from build123d import *

# Parameters (mm, degrees)
F1_DEPTH = 6.35
F0_W     = 265.508406
F0_H     = 162.831157
F2_DEPTH = 5.08


with BuildPart() as f1:
    # F0 (on Front) → F1 (new body, symmetric)
    with BuildSketch(Plane.XZ):
        with BuildLine():
            ThreePointArc((-20.447047, -1.391527), (0, -51.461593), (20.447047, -1.391527))
            ThreePointArc((20.447047, -1.391527), (0, 39.077588), (-20.447047, -1.391527))
        make_face()
        with BuildLine():
            ThreePointArc((15.056898, -1.795547), (0, -47.651593), (-15.056898, -1.795547))
            ThreePointArc((-15.056898, -1.795547), (0, 35.267588), (15.056898, -1.795547))
        make_face(mode=Mode.SUBTRACT)
    extrude(amount=F1_DEPTH, both=True)

    # F0 (on Front) → F2 (join, symmetric)
    with BuildSketch(Plane.XZ):
        with Locations((11.139218, -0.917264)):
            Rectangle(F0_W, F0_H)
        with BuildLine():
            ThreePointArc((-20.447047, -1.391527), (0, 39.077588), (20.447047, -1.391527))
            ThreePointArc((20.447047, -1.391527), (0, -51.461593), (-20.447047, -1.391527))
        make_face(mode=Mode.SUBTRACT)
    extrude(amount=F2_DEPTH, both=True)


solid = f1.part
Input: part model. Units: mm. Frame: model coordinates. A direction names the side the tool comes from. Give positions to 0.01 mm unless a question says otherwise; leave off trailing zeros. Write each loop counter-clockwise with the first axis right and the second up, starting at its lowest first coordinate (ties: lowest second). Pieces come first, ordered by that corner, then holes. Notation, with made-up numbers: M 60.25,-34.75 L 73.25,-34.75 A4 ccw 73.25,-30.75 Z; hole C -9,-33 d9. An arc over 180 degrees is marked long. Write item = value, one per line. Start each with the question number.
1) Reachability of faces 1 (the flat face through (9, 0, -82.333)), 2 (the cylindrical face through (0.784, -5.724, 39.065)), 3 (the cylindrical face through (-0.967, 5.706, -51.446)) from +Z, -Z, +X, -X, +Y, -Y: full face, straight path, thin tool, end or side. Return the list, or none.
2) First-contact query: pin 1 Ø8 at (x, z) = (-76, 22) entering from +Y. Flat tip, straight axial feed; report the tip coordinate or a pass-through.
3) Cut plane D-D on x = -56.5. Return the cut outline in (y, z), then the cut area to 3 significant figures.
4) Material intervals for line 1 along Z through (x, y) = (0, -1.25); line 2 along X through (y, z) = (-5.25, 13); line 3 along Y through (x, z) = (65, 60), sorted ascending. Write a range as [from, to].
5) Draft query along Z for faces 4 (the cylindrical face through (0.784, 5.706, 39.065)), 5 (the cylindrical face through (0.891, -0.089, -47.636)), 6 (the flat face through (-17, 6.35, -3)), 7 (the flat face through (9, 0, 80.498)). Return one class per face: +Z half, -Z half, draft (parallel to the pull), parting line (faces both ways), or undercut.
6) Cut plane C-C on y = -3. Return the cut outline in (x, z), then the cut area to 3 significant figures.
7) Cut plane B-B on z = 25. Return the cut outline in (x, y), then the cut area to 3 significant figures.
8) Cut plane A-A on x = 0. Return the cut outline in (y, z).
Solved:
q1.face_1 = -Z, +X, -X, +Y, -Y
q1.face_2 = -Y
q1.face_3 = +Y
q2.pin_1 = 5.08
q3.outline = M -5.08,-82.33 L 5.08,-82.33 L 5.08,80.5 L -5.08,80.5 Z
q3.area = 1,650 mm2
q4.line_1 = [-82.33, -47.65], [35.27, 80.5]
q4.line_2 = [-25.39, -21.58], [21.58, 25.39]
q4.line_3 = [-5.08, 5.08]
q5.face_4 = undercut
q5.face_5 = undercut
q5.face_6 = draft
q5.face_7 = +Z half
q6.outline = M -121.61,-82.33 L 143.89,-82.33 L 143.89,80.5 L -121.61,80.5 Z; hole M -15.06,-1.8 A25.4 ccw long 15.06,-1.8 A21.59 ccw long Z
q6.area = 40,000 mm2
q7.outline = M -121.61,-5.08 L -22.74,-5.08 L -22.74,-6.35 L -18.38,-6.35 L -18.38,6.35 L -22.74,6.35 L -22.74,5.08 L -121.61,5.08 Z; M 18.38,-6.35 L 22.74,-6.35 L 22.74,-5.08 L 143.89,-5.08 L 143.89,5.08 L 22.74,5.08 L 22.74,6.35 L 18.38,6.35 Z
q7.area = 2,350 mm2
q8.outline = M -6.35,-51.46 L -5.08,-51.46 L -5.08,-82.33 L 5.08,-82.33 L 5.08,-51.46 L 6.35,-51.46 L 6.35,-47.65 L -6.35,-47.65 Z; M -6.35,35.27 L 6.35,35.27 L 6.35,39.08 L 5.08,39.08 L 5.08,80.5 L -5.08,80.5 L -5.08,39.08 L -6.35,39.08 Z
